Can you work these out from the model? Positions are in its coordinate system, mm. Face numbers are marked on the shaded views. Give positions to 0.01 mm unless a question says otherwise; leave off trailing zeros. Write each loop counter-clockwise with the first axis right and the second up, starting at its lowest first coordinate (ties: lowest second). Pieces come first, ordered by that corner, then holes.
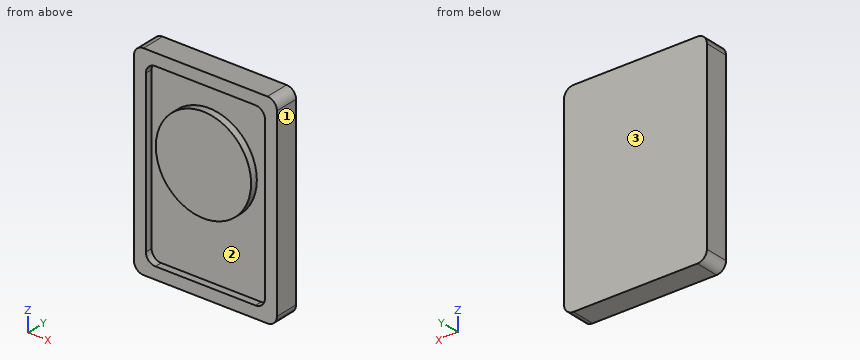
```python
from build123d import *

# Parameters (mm, degrees)
F0_W     = 76.2
F0_H     = 107.95
F1_DEPTH = 12.7
F2_R     = 5.08
F3_W     = 63.5
F3_H     = 95.25
F3_R     = 25.4
F4_DEPTH = 3.81
F5_R     = 5.08


with BuildPart() as f1:
    # F0 (on Front) → F1 (new body)
    with BuildSketch(Plane.XZ):
        with Locations((-9.044009, -26.192475)):
            Rectangle(F0_W, F0_H)
    extrude(amount=F1_DEPTH)

    # F2
    f2_edges = [f1.edges().sort_by_distance(p)[0] for p in [
        (-47.144009, -6.35, 27.782525),
        (29.055991, -6.35, 27.782525),
        (29.055991, -6.35, -80.167475),
        (-47.144009, -6.35, -80.167475),
    ]]
    fillet(f2_edges, radius=F2_R)

    # F3 (on face) → F4 (cut)
    with BuildSketch(Plane.XZ.offset(12.7)):
        with Locations((-9.044009, -26.192475)):
            Rectangle(F3_W, F3_H)
        with Locations((-10.099306, -16.667475)):
            Circle(F3_R, mode=Mode.SUBTRACT)
    extrude(amount=-F4_DEPTH, mode=Mode.SUBTRACT)

    # F5
    f5_edges = [f1.edges().sort_by_distance(p)[0] for p in [
        (-40.794009, -10.795, 21.432525),
        (22.705991, -10.795, 21.432525),
        (22.705991, -10.795, -73.817475),
        (-40.794009, -10.795, -73.817475),
    ]]
    fillet(f5_edges, radius=F5_R)


solid = f1.part
```
1) For pin 1 Ø8 at (x, z) = (-8.5, -48.5) entering from -Y, with a flat end and sliding along its axis, tell me the tip position at first contact or that it passes through.
Values follow:
pin 1: stops at y = -8.89
2) Please list where these lines run through material, in increasing order: L1, parallel to X at y = -10, z = -16; L2, parallel to X at y = -10.5, z = -45; L3, parallel to Z at x = -25.5, y = -11.5.
Values follow:
L1: x = -47.14 to -40.79, -35.49 to 15.29, 22.71 to 29.06
L2: x = -47.14 to -40.79, 22.71 to 29.06
L3: z = -80.17 to -73.82, -36.87 to 3.53, 21.43 to 27.78
3) Suppose I cut it at C-C on x = -8. Write out the boundary of the cut face in (y, z), plus the area to 3 significant figures.
Values follow:
outline: (-12.7, -80.17) - (0, -80.17) - (0, 27.78) - (-12.7, 27.78) - (-12.7, 21.43) - (-8.89, 21.43) - (-8.89, 8.65) - (-12.7, 8.65) - (-12.7, -41.98) - (-8.89, -41.98) - (-8.89, -73.82) - (-12.7, -73.82) - close
area: 1,200 mm2
4) If we mould it in two halves opening along X, with no side actions, what happens to the marked faces 1, 2 and 3? For each: +X half, -X half, draft (parallel to the pull), parting line (faces both ways), or undercut.
Values follow:
face 1: +X half
face 2: undercut
face 3: draft
5) Suppose I cut it at A-A on y = -10. Write out the boundary of the cut face in (x, z).
Values follow:
outline: (-47.14, -75.09) arc R5.08 ccw to (-42.06, -80.17) - (23.98, -80.17) arc R5.08 ccw to (29.06, -75.09) - (29.06, 22.7) arc R5.08 ccw to (23.98, 27.78) - (-42.06, 27.78) arc R5.08 ccw to (-47.14, 22.7) - close; circle Ø50.8 at (-10.1, -16.67); hole (-40.79, -68.74) arc R5.08 ccw to (-35.71, -73.82) - (17.63, -73.82) arc R5.08 ccw to (22.71, -68.74) - (22.71, 16.35) arc R5.08 ccw to (17.63, 21.43) - (-35.71, 21.43) arc R5.08 ccw to (-40.79, 16.35) - close
6) Suppose I cut it at D-D on x = -37. Write out the boundary of the cut face in (y, z), plus the area to 3 significant figures.
Values follow:
outline: (-12.7, -80.17) - (0, -80.17) - (0, 27.78) - (-12.7, 27.78) - (-12.7, 21.27) - (-8.89, 21.27) - (-8.89, -73.65) - (-12.7, -73.65) - close
area: 1,010 mm2
7) Suppose I cut it at B-B on z = -51. Write out the boundary of the cut face in (x, y), plus the area to 3 significant figures.
Values follow:
outline: (-47.14, -12.7) - (-40.79, -12.7) - (-40.79, -8.89) - (22.71, -8.89) - (22.71, -12.7) - (29.06, -12.7) - (29.06, 0) - (-47.14, 0) - close
area: 726 mm2
